```python
from build123d import *

# Parameters (mm, degrees)
F1_DEPTH = 101.6
F2_R     = 3.175
F3_DEPTH = 101.6
F4_R     = 19.05
F5_DEPTH = 38.1


with BuildPart() as f1:
    # F0 (on Top) → F1 (new body)
    with BuildSketch(Plane.XY):
        Polygon((0, 0), (0, 38.1), (-25.4, 38.1), (-25.4, -38.1), (25.4, -38.1), (25.4, 0), align=None)
    extrude(amount=F1_DEPTH)

    # F2 (on face) → F3 (cut, through all)
    with BuildSketch(Plane.XY.offset(101.6)):
        with Locations((-15.875, -28.575)):
            Circle(F2_R)
    extrude(amount=-F3_DEPTH, mode=Mode.SUBTRACT)

    # F4 (on face) → F5 (cut, through all)
    with BuildSketch(Plane.XZ.offset(38.1)):
        with Locations((25.4, 63.5)):
            Circle(F4_R)
    extrude(amount=-F5_DEPTH, mode=Mode.SUBTRACT)


solid = f1.part
```
Read the model definition and answer for the solid it produces. Units are mm, in the model's axes. A direction names the side the tool comes from. Give positions to 0.01 mm unless a question says otherwise; leave off trailing zeros. Write each loop counter-clockwise with the first axis right and the second up, starting at its lowest first coordinate (ties: lowest second). Pieces come first, ordered by that corner, then holes. Notation, with made-up numbers: M 60,21.5 L 113,21.5 A20 cw 113,51.5 Z; hole C -24,85.25 d9. An arc over 180 degrees is marked long. Put each result on its own line as item: value. Start each with the question number.
1. For a pull along Z with two mould halves and no side action, classify faces 3 (the cylindrical face through (-12.847, -27.621, 51.511)), 4 (the flat face through (-6, -8, 0)), 5 (the cylindrical face through (6.355, -19.317, 63.919)), 6 (the flat face through (-6, -8, 101.6)) as released by +Z, released by -Z, zero draft, split by the parting line, or undercut.
2. The part is cut by section D-D, the plane z = 69.5. Give the vertices of the cut face in (x, y) (3 decimals).
3. The part is cut by section B-B, the plane z = 55. Give the vertices of the cut face in (x, y) (3 decimals), and give its area (3 significant figures).
4. Which of the six approach directions +Z, -Z, +X, -X, +Y, -Y give full straight-line access (tool end or side, diameter ignored) to faces 1 (the flat face through (0, 19, 50)), 2 (the flat face through (0, -38.1, 50))?
5. Consider line 1 along X through (y, z) = (16.5, 23); line 2 along Y through (x, z) = (8, 38); line 3 along Y through (x, z) = (-15, 11.5). Determine where each line is inside the solid, lowest interval first.
6. The part is cut by section C-C, the plane x = 2.5. Give the vertices of the cut face in (y, z).
7. Each of these flat-tipped pins is pushed along its axis until it touches: pin 1 Ø7.5 at (x, z) = (13, 34.5) entering from +Y; pin 2 Ø10 at (y, z) = (15.5, 14.5) entering from +X. Where does it stop, or does it pass through?
8. The part is cut by section A-A, the plane x = 11. Give the vertices of the cut face in (y, z), and give its area (3 significant figures).
Final values:
1. face 3: zero draft
1. face 4: released by -Z
1. face 5: undercut
1. face 6: released by +Z
2. outline: M -25.4,-38.1 L 7.32,-38.1 L 7.32,0 L 0,0 L 0,38.1 L -25.4,38.1 Z; hole C -15.875,-28.575 d6.35
3. outline: M -25.4,-38.1 L 8.351,-38.1 L 8.351,0 L 0,0 L 0,38.1 L -25.4,38.1 Z; hole C -15.875,-28.575 d6.35
3. area: 2,220 mm²
4. face 1: +Z, -Z, +X, +Y
4. face 2: +Z, -Z, +X, -X, -Y
5. line 1: x = -25.4 to 0
5. line 2: y = -38.1 to 0
5. line 3: y = -38.1 to -31.63, -25.52 to 38.1
6. outline: M -38.1,0 L 0,0 L 0,101.6 L -38.1,101.6 Z
7. pin 1: stops at y = 0
7. pin 2: stops at x = 0
8. outline: M -38.1,0 L 0,0 L 0,51.03 L -38.1,51.03 Z; M -38.1,75.97 L 0,75.97 L 0,101.6 L -38.1,101.6 Z
8. area: 2,920 mm²
